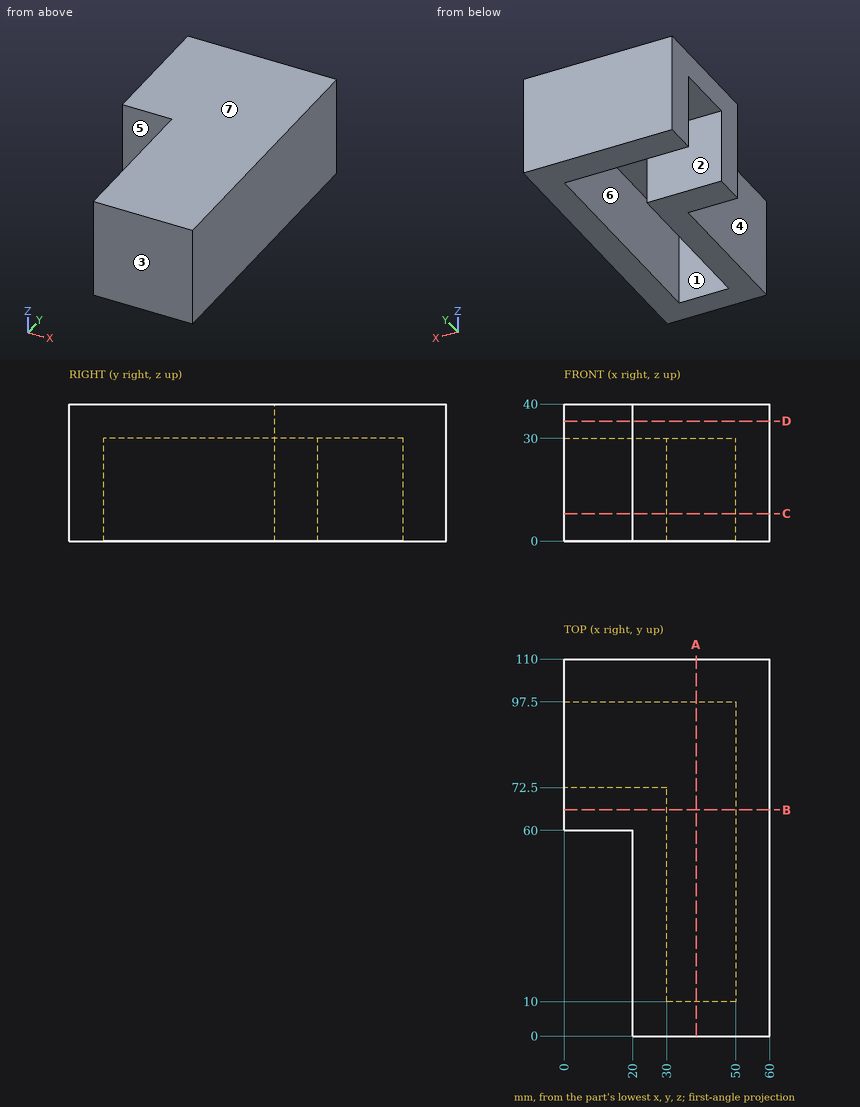
Geometry check sheet. Reference: drawing and pictorial views, mm from the part's lowest x, y, z. A direction names the side the tool comes from. Round coordinates to 2 decimals unless told otherwise and drop trailing zeros. Loops run counter-clockwise (first coordinate to the right, second up) from the corner with the lowest first, then second, coordinate; pieces in that order, holes last. Notation, with made-up numbers: (11, -21) - (20, -21) arc R7 ccw to (20, -9) - close; hole circle Ø6 at (-1, 86.25). An arc over 180 degrees is marked (long way). Answer as CSV lines item,"result".
(1) Cross-section at B-B, the plane y = 66. Enter the section's corners in (x, z), and give its area (3 significant figures).
Output values:
outline,"(0, 0) - (30, 0) - (30, 30) - (50, 30) - (50, 0) - (60, 0) - (60, 40) - (0, 40) - close"
area,"1,800 mm²"
(2) Cross-section at C-C, the plane z = 8. Enter the section's corners in (x, y).
Output values:
outline,"(0, 60) - (20, 60) - (20, 0) - (60, 0) - (60, 110) - (0, 110) - (0, 97.5) - (50, 97.5) - (50, 10) - (30, 10) - (30, 72.5) - (0, 72.5) - close"
(3) Material ranges on line 1 along X through (y, z) = (65, 26); line 2 along Y through (x, z) = (38, 13); line 3 along X through (y, z) = (42.5, 10), recorded low to high.
Output values:
line 1,"x = 0 to 30, 50 to 60"
line 2,"y = 0 to 10, 97.5 to 110"
line 3,"x = 20 to 30, 50 to 60"
(4) Set-up check for the marked faces 1, 2, 3 and 4: record each of +Z, -Z, +X, -X, +Y, -Y from which the full face is reachable in a straight line by a thin tool's end or side.
Output values:
face 1,"-Z"
face 2,"-Z, -X"
face 3,"+Z, -Z, +X, -X, -Y"
face 4,"+Z, -Z, -X, -Y"
(5) Cross-section at A-A, the plane x = 38.5. Enter the section's corners in (y, z).
Output values:
outline,"(0, 0) - (10, 0) - (10, 30) - (97.5, 30) - (97.5, 0) - (110, 0) - (110, 40) - (0, 40) - close"
(6) Cross-section at D-D, the plane z = 35. Enter the section's corners in (x, y).
Output values:
outline,"(0, 60) - (20, 60) - (20, 0) - (60, 0) - (60, 110) - (0, 110) - close"
(7) Depth check by flat-ended pin: pin 1 Ø3 at (x, y) = (23, 76) entering from -Z; pin 2 Ø9 at (x, z) = (15, 21.5) entering from -Y. Enter the tip coordinate at first touch or a pass-through.
Output values:
pin 1,"stops at z = 30"
pin 2,"stops at y = 60"
(8) Release check for a two-part mould opening along Y. For the marked faces 5, 6 and 7 record: released by +Y, released by -Y, zero draft, split by the parting line, or undercut.
Output values:
face 5,"released by -Y"
face 6,"undercut"
face 7,"zero draft"
